Could you check a few things on this model? Use its own coordinates, in mm. A direction names the side the tool comes from. Give positions to 0.01 mm unless a question says otherwise; leave off trailing zeros. Order: outer loops, then holes, each group sorted by start corner. A loop starts at its lowest first (then second) coordinate and runs counter-clockwise, first axis right, second up.
(1) Imagine slicing it at A-A, the plane x = 0. Write out the boundary of the cut face in (y, z).
(2) Will these pins go through, and if not, where does the flat tip stop? pin 1 (6 mm diameter, centred on x = 2.5, y = -29, fed in from +Z); pin 2 (9.5 mm diameter, centred on y = -19, z = 3, fed in from +X); pin 3 (9.5 mm diameter, centred on y = -37, z = 1, fed in from -X); pin 4 (17 mm diameter, centred on x = 7, z = 2.5, fed in from -Y).
(3) Imagine slicing it at C-C, the plane y = -32. Write out the boundary of the cut face in (x, z), then the cut area to 3 significant figures.
(4) If we mould it in two halves opening along Y, with no side actions, what happens to faces 1 (the flat face through (3.75, -27, 0)), 2 (the flat face through (0, 0, 0)), 3 (the cylindrical face through (0.053, -43.327, -1.73))? For each: released by +Y, released by -Y, zero draft, split by the parting line, or undercut.
(5) Imagine slicing it at B-B, the plane z = 0. Write out the boundary of the cut face in (x, y), then the cut area to 3 significant figures.
(6) Imagine slicing it at D-D, the plane x = 11.5. Write out the boundary of the cut face in (y, z), then the cut area to 3 significant figures.
(7) On a 3-axis mill with a long thin cutter (end or side, diameter ignored), from which of +Z, -Z, +X, -X, +Y, -Y can I reach the whole of each face in a straight line? I mean faces 4 (the cylindrical face through (0, -27, -7)), 5 (the cylindrical face through (0, -27, 7)), 6 (the flat face through (0, -50, 0)), 7 (the flat face through (-3.75, -27, 0)), 8 (the cylindrical face through (16.855, -2.465, -2.213)). Say none if no direction works.
(8) If I drill on probe 1 along Y at (x, z) = (1, 0); probe 2 along Y at (x, z) = (-14, -1); probe 3 along X at (y, z) = (-12, 2), over which ranges is the centre line in solid material (lowest first)?
from build123d import *

# Parameters (mm, degrees)
SKETCH1_R           = 17
BOSS_EXTRUDE1_DEPTH = 5
BOSS_EXTRUDE2_START = -5
BOSS_EXTRUDE2_DEPTH = 45
SKETCH2_R           = 3.75
CUT_EXTRUDE1_DEPTH  = 57.741188743


with BuildPart() as part:
    # Sketch1 → Boss-Extrude1 (new body)
    with BuildSketch(Plane(origin=(0, 0, 0), x_dir=(1, 0, 0), z_dir=(0, 1, 0))):
        with Locations(Location((0, 0, 0), (0, 0, 270))):
            Circle(SKETCH1_R)
    extrude(amount=-BOSS_EXTRUDE1_DEPTH)

    # Sketch1<3> → Boss-Extrude2 (add)
    with BuildSketch(Plane(origin=(0, 0, 0), x_dir=(1, 0, 0), z_dir=(0, 1, 0)).offset(BOSS_EXTRUDE2_START)):
        with BuildLine():
            ThreePointArc((-3.75, -5.910795209), (0, -7), (3.75, -5.910795209))
            Line((3.75, -5.910795209), (3.75, 5.910795209))
            ThreePointArc((3.75, 5.910795209), (0, 7), (-3.75, 5.910795209))
            Line((-3.75, 5.910795209), (-3.75, -5.910795209))
        make_face()
    extrude(amount=-BOSS_EXTRUDE2_DEPTH)

    # Sketch2 → Cut-Extrude1 (cut, through all)
    with BuildSketch(Plane(origin=(3.75, 0, 0), x_dir=(0, 0, -1), z_dir=(1, 0, 0))):
        with Locations((0, -40)):
            Circle(SKETCH2_R)
    extrude(amount=-CUT_EXTRUDE1_DEPTH, mode=Mode.SUBTRACT)


solid = part.part
Answer block:
1. outline: (-50, -7) - (-5, -7) - (-5, -17) - (0, -17) - (0, 17) - (-5, 17) - (-5, 7) - (-50, 7) - close; hole circle Ø7.5 at (-40, 0)
2. pin 1: stops at z = 7
2. pin 2: stops at x = 3.75
2. pin 3: stops at x = -3.75
2. pin 4: stops at y = -50
3. outline: (-3.75, -5.91) arc R7 ccw to (3.75, -5.91) - (3.75, 5.91) arc R7 ccw to (-3.75, 5.91) - close
3. area: 99.7 mm2
4. face 1: zero draft
4. face 2: released by +Y
4. face 3: undercut
5. outline: (-17, -5) - (-3.75, -5) - (-3.75, -36.25) - (3.75, -36.25) - (3.75, -5) - (17, -5) - (17, 0) - (-17, 0) - close; (-3.75, -50) - (3.75, -50) - (3.75, -43.75) - (-3.75, -43.75) - close
5. area: 451 mm2
6. outline: (-5, -12.52) - (0, -12.52) - (0, 12.52) - (-5, 12.52) - close
6. area: 125 mm2
7. face 4: -Z, -Y
7. face 5: +Z, -Y
7. face 6: +Z, -Z, +X, -X, -Y
7. face 7: +Z, -Z, -X, -Y
7. face 8: +Y, -Y
8. probe 1: y = -50 to -43.75, -36.25 to 0
8. probe 2: y = -5 to 0
8. probe 3: x = -3.75 to 3.75
